Source: CAD feature listing. Evaluate the final solid. Frame: model axes, mm. A direction names the side the tool comes from. Give positions to 0.01 mm unless a question says otherwise; leave off trailing zeros. Write each loop counter-clockwise with the first axis right and the second up, starting at its lowest first coordinate (ties: lowest second). Pieces come first, ordered by that corner, then holes. Notation, with made-up numbers: M 88.5,34.25 L 114.5,34.25 A22 cw 114.5,73.25 Z; hole C -15.75,-34.75 d11. An arc over 180 degrees is marked long. Use CSV: the item, a comma, the result in double quotes. Start each with the question number.
from build123d import *

# Parameters (mm, degrees)
EXTRUDE_1_DEPTH     = 200
FILLET_1_R          = 8
FILLET_2_R          = 6
SKETCH_2_R          = 1.5
CUT_EXTRUDE_1_DEPTH = 203.484567313
SKETCH_3_W          = 63.1289962
SKETCH_3_H          = 24.316742519
CUT_EXTRUDE_2_DEPTH = 59
CUT_EXTRUDE_START   = -40
CUT_EXTRUDE_3_DEPTH = 40
CUT_EXTRUDE_4_DEPTH = 40


with BuildPart() as part:
    # 草图1 → 凸台-拉伸1 (new body)
    with BuildSketch(Plane.XY):
        Polygon((12, -7), (12, 10), (15, 10), (15, -10), (-15, -10), (-15, 10), (-12, 10), (-12, -7), align=None)
    extrude(amount=EXTRUDE_1_DEPTH)

    # 圆角1
    fillet_1_edges = [part.edges().sort_by_distance(p)[0] for p in [
        (15, -10, 100),
        (-15, -10, 100),
    ]]
    fillet(fillet_1_edges, radius=FILLET_1_R)

    # 圆角2
    fillet_2_edges = [part.edges().sort_by_distance(p)[0] for p in [
        (-12, -7, 100),
        (12, -7, 100),
    ]]
    fillet(fillet_2_edges, radius=FILLET_2_R)

    # 草图2 → 切除-拉伸1 (cut, through all)
    with BuildSketch(Plane.ZY.offset(15)):
        with Locations((90, 5)):
            Circle(SKETCH_2_R)
        with Locations((70, 5)):
            Circle(SKETCH_2_R)
        with Locations((50, 5)):
            Circle(SKETCH_2_R)
        with Locations((30, 5)):
            Circle(SKETCH_2_R)
        with Locations((10, 5)):
            Circle(SKETCH_2_R)
        with Locations(Location((190, 5, 0), (0, 0, 180))):
            Circle(SKETCH_2_R)
        with Locations(Location((170, 5, 0), (0, 0, 180))):
            Circle(SKETCH_2_R)
        with Locations(Location((150, 5, 0), (0, 0, 180))):
            Circle(SKETCH_2_R)
        with Locations(Location((130, 5, 0), (0, 0, 180))):
            Circle(SKETCH_2_R)
        with Locations(Location((110, 5, 0), (0, 0, 180))):
            Circle(SKETCH_2_R)
    extrude(amount=-CUT_EXTRUDE_1_DEPTH, mode=Mode.SUBTRACT)

    # 草图3 → 切除-拉伸2 (cut)
    with BuildSketch(Plane.ZY.offset(15)):
        with Locations((171.5644981, -2.15837126)):
            Rectangle(SKETCH_3_W, SKETCH_3_H)
    extrude(amount=-CUT_EXTRUDE_2_DEPTH, mode=Mode.SUBTRACT)

    # 草图4 → 切除-拉伸3 (cut)
    with BuildSketch(Plane(origin=(0, 0, 0), x_dir=(-1, 0, 0), z_dir=(0, 0, -1)).offset(CUT_EXTRUDE_START)):
        with BuildLine():
            Line((-15, 10), (-15, -2))
            ThreePointArc((-15, -2), (-12.656854249, -7.656854249), (-7, -10))
            Line((-7, -10), (7, -10))
            ThreePointArc((7, -10), (12.656854249, -7.656854249), (15, -2))
            Line((15, -2), (15, 10))
            Line((15, 10), (12, 10))
            Line((12, 10), (12, -1))
            ThreePointArc((12, -1), (10.242640687, -5.242640687), (6, -7))
            Line((6, -7), (-6, -7))
            ThreePointArc((-6, -7), (-10.242640687, -5.242640687), (-12, -1))
            Line((-12, -1), (-12, 10))
            Line((-12, 10), (-15, 10))
        make_face()
    extrude(amount=CUT_EXTRUDE_3_DEPTH, mode=Mode.SUBTRACT)

    # 草图5 → 切除-拉伸4 (cut)
    with BuildSketch(Plane.XY.offset(140)):
        with BuildLine():
            Line((15, 10), (12, 10))
            Line((12, 10), (12, -1))
            ThreePointArc((12, -1), (10.242640687, -5.242640687), (6, -7))
            Line((6, -7), (-6, -7))
            ThreePointArc((-6, -7), (-10.242640687, -5.242640687), (-12, -1))
            Line((-12, -1), (-12, 10))
            Line((-12, 10), (-15, 10))
            Line((-15, 10), (-15, -2))
            ThreePointArc((-15, -2), (-12.656854249, -7.656854249), (-7, -10))
            Line((-7, -10), (7, -10))
            ThreePointArc((7, -10), (12.656854249, -7.656854249), (15, -2))
            Line((15, -2), (15, 10))
        make_face()
    extrude(amount=-CUT_EXTRUDE_4_DEPTH, mode=Mode.SUBTRACT)


solid = part.part
Item 1: Section D-D (z = 95). Return the cut outline in (x, y).
Item 2: Material intervals for probe 1 along X at (y, z) = (1, 49.5); probe 2 along Y at (x, z) = (-1.5, 64); probe 3 along Y at (x, z) = (13.75, 70), sorted ascending.
Item 3: Pull-direction query (Z, two-part tool) for faces 1 (the flat face through (-0.1, -7.4, 100)), 2 (the flat face through (0.1, -7.4, 40)), 3 (the flat face through (-12, 3, 70)), 4 (the cylindrical face through (-13.52, 5.45, 91.43)); classes: released by +Z, released by -Z, zero draft, split by the parting line, or undercut.
Item 4: Section B-B (z = 50). Return the cut outline in (x, y), plus the area to 3 significant figures.
Item 5: Section A-A (y = 8.25). Return the cut outline in (x, z).
Item 6: Contact query for flat-ended pins moving along their axis: pin 1 Ø2 at (y, z) = (-3.5, 62) entering from +X; pin 2 Ø1 at (x, z) = (11.5, 67.5) entering from -Y; pin 3 Ø13 at (x, z) = (-3, 64.5) entering from +Y. Output: stop coordinate, or through.
Item 7: Set-up query: faces 5 (the cylindrical face through (13.48, 5.45, 91.43)), 6 (the flat face through (0, -7, 70)). Return all of +Z, -Z, +X, -X, +Y, -Y with unobstructed straight access to the full face (end or side cutting, diameter ignored); none if empty.
Item 8: Section C-C (y = 5). State how many separate pieces and enclosed holes the cut face has, plus the area to 3 significant figures.
Output values:
1,outline,"M -15,-2 A8 ccw -7,-10 L 7,-10 A8 ccw 15,-2 L 15,10 L 12,10 L 12,-1 A6 cw 6,-7 L -6,-7 A6 cw -12,-1 L -12,10 L -15,10 Z"
2,probe 1,"x = -15 to -12, 12 to 15"
2,probe 2,"y = -10 to -7"
2,probe 3,"y = -6.29 to 3.5, 6.5 to 10"
3,face 1,"released by +Z"
3,face 2,"released by -Z"
3,face 3,"zero draft"
3,face 4,"undercut"
4,outline,"M -15,-2 A8 ccw -7,-10 L 7,-10 A8 ccw 15,-2 L 15,3.5 L 12,3.5 L 12,-1 A6 cw 6,-7 L -6,-7 A6 cw -12,-1 L -12,3.5 L -15,3.5 Z; M -15,6.5 L -12,6.5 L -12,10 L -15,10 Z; M 12,6.5 L 15,6.5 L 15,10 L 12,10 Z"
4,area,"162 mm2"
5,outline,"M -15,40 L -12,40 L -12,100 L -15,100 Z; M 12,40 L 15,40 L 15,100 L 12,100 Z"
6,pin 1,"stops at x = 14.98"
6,pin 2,"stops at y = -8.93"
6,pin 3,"stops at y = -5.87"
7,face 5,"+X, -X"
7,face 6,"+Z, -Z, +Y"
8,separate pieces,"8"
8,enclosed holes,"0"
8,area,"306 mm2"
